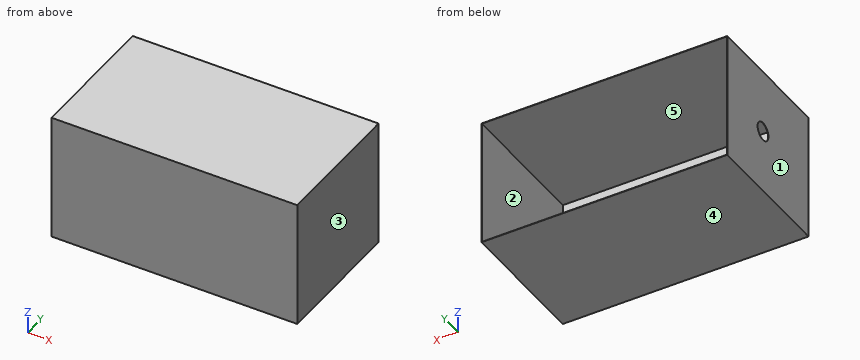
```python
from build123d import *

# Parameters (mm, degrees)
MASTER_FOOTPRINT_W    = 1350
MASTER_FOOTPRINT_H    = 700
BATH_BASE_PLATE_DEPTH = 750
BATH_SHELL_2MM_T      = -2
SKETCH_1_R            = 50
INLET_D100_CUT_DEPTH  = 10


with BuildPart() as part:
    # MASTER_FOOTPRINT → BATH_BASE_PLATE (new body)
    with BuildSketch(Plane(origin=(0, 0, 0), x_dir=(1, 0, 0), z_dir=(0, 1, 0))):
        with Locations((675, 350)):
            Rectangle(MASTER_FOOTPRINT_W, MASTER_FOOTPRINT_H)
    extrude(amount=BATH_BASE_PLATE_DEPTH)

    # BATH_SHELL_2MM
    bath_shell_2mm_openings = [part.faces().sort_by_distance(p)[0] for p in [
        (675, 750, -350),
    ]]
    offset(amount=BATH_SHELL_2MM_T, openings=bath_shell_2mm_openings, kind=Kind.INTERSECTION)

    # Эскиз1 → INLET_D100_CUT (cut)
    with BuildSketch(Plane(origin=(0, 0, 0), x_dir=(0, 0, -1), z_dir=(1, 0, 0))):
        with Locations((350, 420)):
            Circle(SKETCH_1_R)
    extrude(amount=INLET_D100_CUT_DEPTH, mode=Mode.SUBTRACT)


solid = part.part
```
Geometry check sheet. Reference: the model listing, model coordinates, mm. Face numbers are marked on the shaded views. A direction names the side the tool comes from. Round coordinates to 2 decimals unless told otherwise and drop trailing zeros. Order: outer loops, then holes, each group sorted by start corner. A loop starts at its lowest first (then second) coordinate and runs counter-clockwise, first axis right, second up. Notation, with made-up numbers: (53.5, 34.25) - (83.5, 34.25) arc R13 cw to (83.5, 56.25) - close; hole circle Ø7 at (66, 33). An arc over 180 degrees is marked (long way). Use a Markdown table: item, result. Add a question column.
1) Mould release check, pull along X, two halves, no side actions. Record for the marked faces 3, 4 and 5: released by +X, released by -X, zero draft, split by the parting line, or undercut.
2) Thickness scan on line 1 along Z through (x, y) = (1, 420); line 2 along X through (y, z) = (361.5, -530); line 3 along Z through (x, y) = (1104.5, 704.5). Record the ranges inside material, lowest first.
3) Section check C-C (y = 420). Record the cut outline in (x, z).
4) Gauge pin test, flat ends, axial feed: P1, Ø3, axis at y = 85, z = -573, coming from the -X side; P2, Ø5, axis at x = 912.5, z = -321, coming from the +Y side. Record the tip position at first contact, or that the pin passes through.
5) Section check B-B (y = 661). Record the cut outline in (x, z).
6) Section check A-A (z = -350). Record the cut outline in (x, y), then the cut area to 3 significant figures.
7) Set-up check for the marked faces 1 and 2: record each of +Z, -Z, +X, -X, +Y, -Y from which the full face is reachable in a straight line by a thin tool's end or side.
8) Section check D-D (z = -253). Record the cut outline in (x, y).
Established:
| question | item | result |
|---|---|---|
| 1 | face 3 | released by +X |
| 1 | face 4 | zero draft |
| 1 | face 5 | undercut |
| 2 | line 1 | -700 to -400, -300 to 0 |
| 2 | line 2 | 0 to 2, 1348 to 1350 |
| 2 | line 3 | -700 to -698, -2 to 0 |
| 3 | outline | (0, -700) - (1350, -700) - (1350, 0) - (0, 0) - (0, -300) - (2, -300) - (2, -2) - (1348, -2) - (1348, -698) - (2, -698) - (2, -400) - (0, -400) - close |
| 4 | P1 | x = 0 |
| 4 | P2 | y = 2 |
| 5 | outline | (0, -700) - (1350, -700) - (1350, 0) - (0, 0) - close; hole (2, -698) - (1348, -698) - (1348, -2) - (2, -2) - close |
| 6 | outline | (0, 0) - (1350, 0) - (1350, 750) - (1348, 750) - (1348, 2) - (2, 2) - (2, 370) - (0, 370) - close; (0, 470) - (2, 470) - (2, 750) - (0, 750) - close |
| 6 | area | 5,490 mm2 |
| 7 | face 1 | +Z, -Z, -X, +Y, -Y |
| 7 | face 2 | +Y |
| 8 | outline | (0, 0) - (1350, 0) - (1350, 750) - (1348, 750) - (1348, 2) - (2, 2) - (2, 750) - (0, 750) - close |
